Could you check a few things on this model? Use its own coordinates, in mm. A direction names the side the tool comes from. Coordinates: 2 decimals unless noted, no trailing zeros. Write each loop counter-clockwise with the first axis right and the second up, starting at its lowest first coordinate (ties: lowest second). Pieces come first, ordered by that corner, then holes.
```python
from build123d import *

# Parameters (mm, degrees)
SKETCH1_W               = 40.35
SKETCH1_H               = 43.35
BOSS_EXTRUDE1_DEPTH     = 47
CUT_EXTRUDE2_DEPTH      = 102
FILLET1_R               = 10
CUT_EXTRUDE3_DEPTH      = 102
FILLET2_R               = 5
CUT_EXTRUDE4_DEPTH      = 102
CUT_EXTRUDE4_DEPTH_BACK = 102
SKETCH6_R               = 1.73
CUT_EXTRUDE5_DEPTH      = 102
SKETCH8_R               = 1.55
CUT_EXTRUDE6_DEPTH      = 102
SKETCH9_R               = 1.75
CUT_EXTRUDE7_DEPTH      = 10


with BuildPart() as part:
    # Sketch1 → Boss-Extrude1 (new body)
    with BuildSketch(Plane(origin=(0, 0, 0), x_dir=(1, 0, 0), z_dir=(0, 1, 0))):
        with Locations((-26.966212793, -29.108023223)):
            Rectangle(SKETCH1_W, SKETCH1_H)
    extrude(amount=BOSS_EXTRUDE1_DEPTH)

    # Sketch3 → Cut-Extrude2 (cut)
    with BuildSketch(Plane.XY.offset(50.783023223)):
        with BuildLine():
            Line((-47.141212793, 47), (-47.141212793, 26.825))
            ThreePointArc((-47.141212793, 26.825), (-41.232092103, 41.09087931), (-26.966212793, 47))
            Line((-26.966212793, 47), (-47.141212793, 47))
        make_face()
        with BuildLine():
            Line((-6.791212793, 47), (-26.966212793, 47))
            ThreePointArc((-26.966212793, 47), (-12.700333482, 41.09087931), (-6.791212793, 26.825))
            Line((-6.791212793, 26.825), (-6.791212793, 47))
        make_face()
    extrude(amount=-CUT_EXTRUDE2_DEPTH, mode=Mode.SUBTRACT)

    # Fillet1
    fillet1_edges = [part.edges().sort_by_distance(p)[0] for p in [
        (-26.966212793, 0, 50.783023223),
    ]]
    fillet(fillet1_edges, radius=FILLET1_R)

    # Sketch5 → Cut-Extrude3 (cut)
    with BuildSketch(Plane.ZY.offset(47.141212793)):
        with BuildLine():
            Line((-6.665763497, 3.45), (36.595559978, 3.45))
            Line((36.595559978, 3.45), (40.783023223, 3.45))
            ThreePointArc((40.783023223, 3.45), (45.41457264, 5.368450583), (47.333023223, 10))
            Line((47.333023223, 10), (47.333023223, 17.578484004))
            Line((47.333023223, 17.578484004), (47.333023223, 59.778436909))
            Line((47.333023223, 59.778436909), (-6.665763497, 59.778436909))
            Line((-6.665763497, 59.778436909), (-6.665763497, 3.45))
        make_face()
    extrude(amount=-CUT_EXTRUDE3_DEPTH, mode=Mode.SUBTRACT)

    # Fillet2
    fillet2_edges = [part.edges().sort_by_distance(p)[0] for p in [
        (-6.791212793, 1.725, 7.433023223),
        (-47.141212793, 1.725, 7.433023223),
    ]]
    fillet(fillet2_edges, radius=FILLET2_R)

    # Sketch6 → Cut-Extrude4 (cut, two sides: drawn at the far end of the back side and taken through both)
    with BuildSketch(Plane(origin=(0, 3.45, 0), x_dir=(1, 0, 0), z_dir=(0, 1, 0)).offset(-CUT_EXTRUDE4_DEPTH_BACK)):
        with BuildLine():
            Line((-10.653989329, -40.783023223), (-13.388436256, -40.783023223))
            ThreePointArc((-13.388436256, -40.783023223), (-12.021212793, -41.453023223), (-10.653989329, -40.783023223))
        make_face()
        with BuildLine():
            ThreePointArc((-12.021212793, -37.993023223), (-13.57470885, -38.961741409), (-13.388436256, -40.783023223))
            Line((-13.388436256, -40.783023223), (-10.653989329, -40.783023223))
            ThreePointArc((-10.653989329, -40.783023223), (-10.384417663, -40.283203287), (-10.291212793, -39.723023223))
            ThreePointArc((-10.291212793, -39.723023223), (-10.797918061, -38.499728491), (-12.021212793, -37.993023223))
        make_face()
        with BuildLine():
            ThreePointArc((-41.911212793, -37.993023223), (-43.134507524, -38.499728491), (-43.641212793, -39.723023223))
            ThreePointArc((-43.641212793, -39.723023223), (-43.548007922, -40.283203287), (-43.278436256, -40.783023223))
            Line((-43.278436256, -40.783023223), (-40.543989329, -40.783023223))
            ThreePointArc((-40.543989329, -40.783023223), (-40.274417663, -40.283203287), (-40.181212793, -39.723023223))
            ThreePointArc((-40.181212793, -39.723023223), (-40.687918061, -38.499728491), (-41.911212793, -37.993023223))
        make_face()
        with BuildLine():
            Line((-40.543989329, -40.783023223), (-43.278436256, -40.783023223))
            ThreePointArc((-43.278436256, -40.783023223), (-41.911212793, -41.453023223), (-40.543989329, -40.783023223))
        make_face()
        with Locations(Location((-12.021212793, -15.663023223, 0), (0, 0, 90))):
            Circle(SKETCH6_R)
        with Locations(Location((-41.911212793, -15.663023223, 0), (0, 0, 90))):
            Circle(SKETCH6_R)
    extrude(amount=CUT_EXTRUDE4_DEPTH + CUT_EXTRUDE4_DEPTH_BACK, mode=Mode.SUBTRACT)

    # Sketch7 → Cut-Extrude5 (cut)
    with BuildSketch(Plane.XY.offset(50.783023223)):
        with BuildLine():
            Line((-33.541212793, 33.925), (-33.541212793, 19.945))
            ThreePointArc((-33.541212793, 19.945), (-26.966212793, 13.37), (-20.391212793, 19.945))
            Line((-20.391212793, 19.945), (-20.391212793, 33.925))
            ThreePointArc((-20.391212793, 33.925), (-26.966212793, 40.5), (-33.541212793, 33.925))
        make_face()
    extrude(amount=-CUT_EXTRUDE5_DEPTH, mode=Mode.SUBTRACT)

    # Sketch8 → Cut-Extrude6 (cut)
    with BuildSketch(Plane.XY.offset(50.783023223)):
        with Locations((-34.766212793, 13.372769702)):
            Circle(SKETCH8_R)
        with Locations((-19.166212793, 13.372769702)):
            Circle(SKETCH8_R)
        with BuildLine():
            ThreePointArc((-12.966212793, 26.825), (-11.416212793, 25.275), (-9.866212793, 26.825))
            Line((-9.866212793, 26.825), (-12.966212793, 26.825))
        make_face()
        with BuildLine():
            Line((-12.966212793, 26.825), (-9.866212793, 26.825))
            ThreePointArc((-9.866212793, 26.825), (-11.416212793, 28.375), (-12.966212793, 26.825))
        make_face()
        with BuildLine():
            ThreePointArc((-44.066212793, 26.825), (-42.516212793, 25.275), (-40.966212793, 26.825))
            Line((-40.966212793, 26.825), (-44.066212793, 26.825))
        make_face()
        with BuildLine():
            Line((-44.066212793, 26.825), (-40.966212793, 26.825))
            ThreePointArc((-40.966212793, 26.825), (-42.516212793, 28.375), (-44.066212793, 26.825))
        make_face()
        with Locations((-34.766212793, 40.277230298)):
            Circle(SKETCH8_R)
        with Locations((-19.166212793, 40.277230298)):
            Circle(SKETCH8_R)
    extrude(amount=-CUT_EXTRUDE6_DEPTH, mode=Mode.SUBTRACT)

    # Sketch9 → Cut-Extrude7 (cut)
    with BuildSketch(Plane.XZ):
        with Locations(Location((-26.911212793, 15.483023223, 0), (0, 0, 270))):
            Circle(SKETCH9_R)
    extrude(amount=-CUT_EXTRUDE7_DEPTH, mode=Mode.SUBTRACT)


solid = part.part
```
1. For pin 1 (1.7 mm diameter, centred on y = 29.5, z = 48.5, fed in from +X); pin 2 (5 mm diameter, centred on x = -29, y = 13, fed in from -Z); pin 3 (12 mm diameter, centred on x = -18, z = 34.5, fed in from +Y), each with a flat end and sliding along its axis, tell me the tip position at first contact or that it passes through.
Verdict:
pin 1: stops at x = -6.87
pin 2: stops at z = 47.33
pin 3: stops at y = 3.45
2. Please list where these lines run through material, in increasing order: line 1 along Z through (x, y) = (-16, 17.5); line 2 along Y through (x, z) = (-39, 17); line 3 along X through (y, z) = (36, 49).
Verdict:
line 1: z = 47.33 to 50.78
line 2: y = 0 to 3.45
line 3: x = -44.93 to -33.21, -20.73 to -9
3. I want a section at C-C on x = -34.5. Please give me the cut outline in (y, z), plus the area to 3 significant figures.
Verdict:
outline: (0, 7.43) - (3.45, 7.43) - (3.45, 40.78) arc R6.55 cw to (10, 47.33) - (11.85, 47.33) - (11.85, 50.78) - (10, 50.78) arc R10 ccw to (0, 40.78) - close; (14.9, 47.33) - (38.75, 47.33) - (38.75, 50.78) - (14.9, 50.78) - close; (41.8, 47.33) - (45.54, 47.33) - (45.54, 50.78) - (41.8, 50.78) - close
area: 261 mm2
4. I want a section at D-D on z = 22. Please give me the cut outline in (x, y).
Verdict:
outline: (-47.14, 0) - (-6.79, 0) - (-6.79, 3.45) - (-47.14, 3.45) - close
5. I want a section at A-A on y = 22.5. Please give me the cut outline in (x, z).
Verdict:
outline: (-47.14, 47.33) - (-33.54, 47.33) - (-33.54, 50.78) - (-47.14, 50.78) - close; (-20.39, 47.33) - (-6.79, 47.33) - (-6.79, 50.78) - (-20.39, 50.78) - close
6. I want a section at B-B on x = -24. Please give me the cut outline in (y, z).
Verdict:
outline: (0, 7.43) - (3.45, 7.43) - (3.45, 40.78) arc R6.55 cw to (10, 47.33) - (14.08, 47.33) - (14.08, 50.78) - (10, 50.78) arc R10 ccw to (0, 40.78) - close; (39.79, 47.33) - (46.78, 47.33) - (46.78, 50.78) - (39.79, 50.78) - close
7. On a 3-axis mill with a long thin cutter (end or side, diameter ignored), from which of +Z, -Z, +X, -X, +Y, -Y can I reach the whole of each face in a straight line? I mean faces 4 (the face through (-33.541, 27, 49)), 5 (the face through (-27, 2, 7.433)), 6 (the face through (-27, 3.45, 24)). Say none if no direction works.
Verdict:
face 4: +Z, -Z
face 5: -Z, +X, -X, +Y, -Y
face 6: -Z, +X, -X, +Y
8. If we mould it in two halves opening along X, with no side actions, what happens to faces 1 (the face through (-18, 28, 47.333)), 2 (the face through (-47.141, 3, 37)), 3 (the face through (-12.646, 25.882, 49.082))? For each: pulls with the +X half, pulls with the -X half, needs draft (parallel to the pull), parting line crosses it, or undercut.
Verdict:
face 1: needs draft
face 2: pulls with the -X half
face 3: undercut
